Can you work these out from the model? Positions are in its coordinate system, mm. Coordinates: 2 decimals unless noted, no trailing zeros. Order: outer loops, then holes, each group sorted by start corner. A loop starts at its lowest first (then second) coordinate and runs counter-clockwise, first axis right, second up. Notation, with made-up numbers: (1, 74.5) -> (52, 74.5) arc R9 cw to (52, 86.5) -> close; hole circle Ø8 at (56, 43.5). An arc over 180 degrees is marked (long way). Use a Markdown table: item, result. Add a question column.
1. If I drill on line 1 along X through (y, z) = (1.05, 29); line 2 along X through (y, z) = (0.8, -52); line 3 along Z through (x, y) = (-51, 0.5), over which ranges is the centre line in solid material (lowest first)? Write a range as from..to.
2. Suppose I cut it at B-B, the plane z = 48. List the corners of the cut face in (x, y) for me.
3. We'd pull the mould along Z, two halves only. Please class faces 1 (the cylindrical face through (-0.08, 0.86, -66.19)), 2 (the cylindrical face through (-65.075, 0.862, 12.104)): pulls with the +Z half, pulls with the -Z half, needs draft (parallel to the pull), parting line crosses it, or undercut.
4. Suppose I cut it at A-A, the plane z = 4.5. List the corners of the cut face in (x, y) for me, then the cut area to 3 significant figures.
5. For pin 1 Ø1 at (x, y) = (-11, 0.5) entering from +Z, with a flat end and sliding along its axis, tell me the tip position at first contact or that it passes through.
6. Suppose I cut it at C-C, the plane y = 0.5. State how many separate pieces and enclosed holes the cut face has, then the cut area to 3 significant figures.
```python
from build123d import *

# Parameters (mm, degrees)
SKETCH1_R           = 70
SKETCH1_R_2         = 50
BOSS_EXTRUDE1_DEPTH = 1.7
SKETCH3_R           = 3.81
CUT_EXTRUDE1_DEPTH  = 2.54
CIRPATTERN1_COUNT   = 43
SKETCH5_R           = 2.5
CUT_EXTRUDE2_DEPTH  = 10


with BuildPart() as part:
    # Sketch1 → Boss-Extrude1 (new body)
    with BuildSketch(Plane(origin=(0, 0, 0), x_dir=(1, 0, 0), z_dir=(0, 1, 0))):
        with Locations(Location((0, 0, 0), (0, 0, 270))):
            Circle(SKETCH1_R)
        with Locations(Location((0, 0, 0), (0, 0, 270))):
            Circle(SKETCH1_R_2, mode=Mode.SUBTRACT)
    extrude(amount=BOSS_EXTRUDE1_DEPTH)

    # Sketch3 → Cut-Extrude1 (cut)
    with BuildSketch(Plane(origin=(0, 1.7, 0), x_dir=(1, 0, 0), z_dir=(0, 1, 0))):
        with Locations((0, 70)):
            Circle(SKETCH3_R)
    cut_extrude1 = extrude(amount=-CUT_EXTRUDE1_DEPTH, mode=Mode.SUBTRACT)

    # CirPattern1: Cut-Extrude1 ×43 about axis
    cirpattern1_axis = Axis((0, 0, 0), (0, 1, 0))
    for i in range(1, CIRPATTERN1_COUNT):
        add(cut_extrude1.rotate(cirpattern1_axis, i * 360 / CIRPATTERN1_COUNT), mode=Mode.SUBTRACT)

    # Sketch5 → Cut-Extrude2 (cut)
    with BuildSketch(Plane(origin=(0, 0, 0), x_dir=(-1, 0, 0), z_dir=(0, -1, 0))):
        with Locations(Location((0, 59.449975509, 0), (0, 0, 90))):
            Circle(SKETCH5_R)
        with Locations(Location((51.485189045, 29.724987755, 0), (0, 0, 90))):
            Circle(SKETCH5_R)
        with Locations(Location((51.485189045, -29.724987755, 0), (0, 0, 90))):
            Circle(SKETCH5_R)
        with Locations(Location((0, -59.449975509, 0), (0, 0, 90))):
            Circle(SKETCH5_R)
        with Locations(Location((-51.485189045, -29.724987755, 0), (0, 0, 90))):
            Circle(SKETCH5_R)
        with Locations(Location((-51.485189045, 29.724987755, 0), (0, 0, 90))):
            Circle(SKETCH5_R)
    extrude(amount=-CUT_EXTRUDE2_DEPTH, mode=Mode.SUBTRACT)


solid = part.part
```
Worked out:
| question | item | result |
|---|---|---|
| 1 | line 1 | x = -59.91..-53.88, -49.09..-40.73, 40.73..49.09, 53.88..59.91 |
| 1 | line 2 | x = -42.9..42.9 |
| 1 | line 3 | z = -47.95..-47.36, -42.2..-32.18, -27.27..27.27, 32.18..44.82 |
| 2 | outline | (-46.63, 0) -> (-14, 0) -> (-14, 1.7) -> (-46.63, 1.7) -> close; (14, 0) -> (46.63, 0) -> (46.63, 1.7) -> (14, 1.7) -> close |
| 3 | face 1 | pulls with the -Z half |
| 3 | face 2 | undercut |
| 4 | outline | (-66.68, 0) -> (-49.8, 0) -> (-49.8, 1.7) -> (-66.68, 1.7) -> close; (49.8, 0) -> (66.68, 0) -> (66.68, 1.7) -> (49.8, 1.7) -> close |
| 4 | area | 57.4 mm² |
| 5 | pin 1 | stops at z = 69.21 |
| 6 | separate pieces | 1 |
| 6 | enclosed holes | 7 |
| 6 | area | 6,450 mm² |
